from build123d import *

# Parameters (mm, degrees)
SKETCH1_W             = 342.9
SKETCH1_H             = 228.6
MAIN_BOX_DEPTH        = 152.4
SHELL1_T              = 6.35
TOP_HOLE_REACH        = 154.4
SKETCH2_R             = 44.45
SIDE_HOLE_REACH       = 344.9
SKETCH3_R             = 44.45
POWER_CORD_HOLE_REACH = 344.9
SKETCH4_W             = 25.4
SKETCH4_H             = 25.4


with BuildPart() as part:
    # Sketch1 → main box (new body)
    with BuildSketch(Plane(origin=(0, 0, 0), x_dir=(1, 0, 0), z_dir=(0, 1, 0))):
        with Locations((171.45, 114.3)):
            Rectangle(SKETCH1_W, SKETCH1_H)
    extrude(amount=MAIN_BOX_DEPTH)

    # Shell1 (no face opened: a closed hollow body)
    add(offset(amount=-SHELL1_T, mode=Mode.PRIVATE), mode=Mode.SUBTRACT)

    # Sketch2 → top hole (cut, up to next)
    with BuildSketch(Plane(origin=(0, 152.4, 0), x_dir=(1, 0, 0), z_dir=(0, 1, 0)), mode=Mode.PRIVATE) as top_hole_sk1:
        with Locations((279.4, 114.3)):
            Circle(SKETCH2_R)
    top_hole_tool1 = extrude(top_hole_sk1.sketch, amount=-TOP_HOLE_REACH, mode=Mode.PRIVATE) & part.part
    add(top_hole_tool1.solids().sort_by_distance((279.4, 152.4, -114.3))[0], mode=Mode.SUBTRACT)

    # Sketch3 → side hole (cut, up to next)
    with BuildSketch(Plane.ZY, mode=Mode.PRIVATE) as side_hole_sk1:
        with Locations((-114.3, 76.2)):
            Circle(SKETCH3_R)
    side_hole_tool1 = extrude(side_hole_sk1.sketch, amount=-SIDE_HOLE_REACH, mode=Mode.PRIVATE) & part.part
    add(side_hole_tool1.solids().sort_by_distance((0, 76.2, -114.3))[0], mode=Mode.SUBTRACT)

    # Sketch4 → power cord hole (cut, up to next)
    with BuildSketch(Plane(origin=(342.9, 0, 0), x_dir=(0, 0, -1), z_dir=(1, 0, 0)), mode=Mode.PRIVATE) as power_cord_hole_sk1:
        with Locations((50.8, 25.4)):
            Rectangle(SKETCH4_W, SKETCH4_H)
    power_cord_hole_tool1 = extrude(power_cord_hole_sk1.sketch, amount=-POWER_CORD_HOLE_REACH, mode=Mode.PRIVATE) & part.part
    add(power_cord_hole_tool1.solids().sort_by_distance((342.9, 25.4, -50.8))[0], mode=Mode.SUBTRACT)


solid = part.part
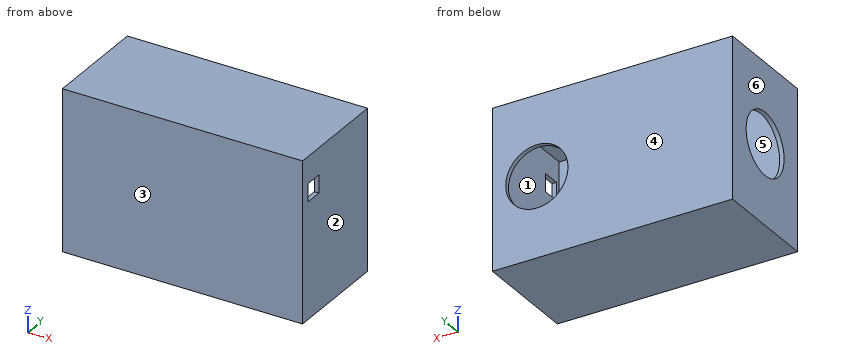
Build history of the part. All positions in model axes, mm. Face numbers are marked on the shaded views. A direction names the side the tool comes from. Give positions to 0.01 mm unless a question says otherwise; leave off trailing zeros. Loops run counter-clockwise (first coordinate to the right, second up) from the corner with the lowest first, then second, coordinate; pieces in that order, holes last. Notation, with made-up numbers: (16.25, -32.75) -> (59.25, -32.75) arc R21 ccw to (59.25, -13.75) -> close; hole circle Ø5 at (83, 29.25). An arc over 180 degrees is marked (long way). Answer in a Markdown table with one row per item.
Item 1: Slice it at B-B on y = 140. Write the cut outline in (x, z), plus the area to 3 significant figures.
Findings below:
| item | result |
|---|---|
| outline | (0, -228.6) -> (342.9, -228.6) -> (342.9, 0) -> (0, 0) -> close; hole (6.35, -222.25) -> (336.55, -222.25) -> (336.55, -6.35) -> (6.35, -6.35) -> close |
| area | 7,100 mm² |
Item 2: Slice it at A-A on z = -114.3. Write the cut outline in (x, y).
Findings below:
| item | result |
|---|---|
| outline | (0, 0) -> (342.9, 0) -> (342.9, 152.4) -> (323.85, 152.4) -> (323.85, 146.05) -> (336.55, 146.05) -> (336.55, 6.35) -> (6.35, 6.35) -> (6.35, 31.75) -> (0, 31.75) -> close; (0, 120.65) -> (6.35, 120.65) -> (6.35, 146.05) -> (234.95, 146.05) -> (234.95, 152.4) -> (0, 152.4) -> close |
Item 3: Tool access for the marked faces 5 and 6: list every direction of +Z, -Z, +X, -X, +Y, -Y with a clear straight run to the whole face (end or side of a thin tool).
Findings below:
| item | result |
|---|---|
| face 5 | none |
| face 6 | +Z, -Z, -X, +Y, -Y |
Item 4: Probe line 1 along Z through (x, y) = (279.4, 150.5); line 2 along Y through (x, z) = (190.5, -97); line 3 along Z through (x, y) = (252.5, 97). List the from-to ranges inside material, lowest first. Write a range as [from, to].
Findings below:
| item | result |
|---|---|
| line 1 | z = [-228.6, -158.75], [-69.85, 0] |
| line 2 | y = [0, 6.35], [146.05, 152.4] |
| line 3 | z = [-228.6, -222.25], [-6.35, 0] |
Item 5: Slice it at C-C on z = -17. Write the cut outline in (x, y), plus the area to 3 significant figures.
Findings below:
| item | result |
|---|---|
| outline | (0, 0) -> (342.9, 0) -> (342.9, 152.4) -> (0, 152.4) -> close; hole (6.35, 6.35) -> (336.55, 6.35) -> (336.55, 146.05) -> (6.35, 146.05) -> close |
| area | 6,130 mm² |
Item 6: Slice it at D-D on x = 279.4. Write the cut outline in (y, z).
Findings below:
| item | result |
|---|---|
| outline | (0, -228.6) -> (152.4, -228.6) -> (152.4, -158.75) -> (146.05, -158.75) -> (146.05, -222.25) -> (6.35, -222.25) -> (6.35, -6.35) -> (146.05, -6.35) -> (146.05, -69.85) -> (152.4, -69.85) -> (152.4, 0) -> (0, 0) -> close |
Item 7: Mould opens along Y. For the marked faces 1, 2, 3 and 4 say: pulls with the +Y half, pulls with the -Y half, needs draft (parallel to the pull), parting line crosses it, or undercut.
Findings below:
| item | result |
|---|---|
| face 1 | undercut |
| face 2 | needs draft |
| face 3 | pulls with the -Y half |
| face 4 | pulls with the +Y half |
